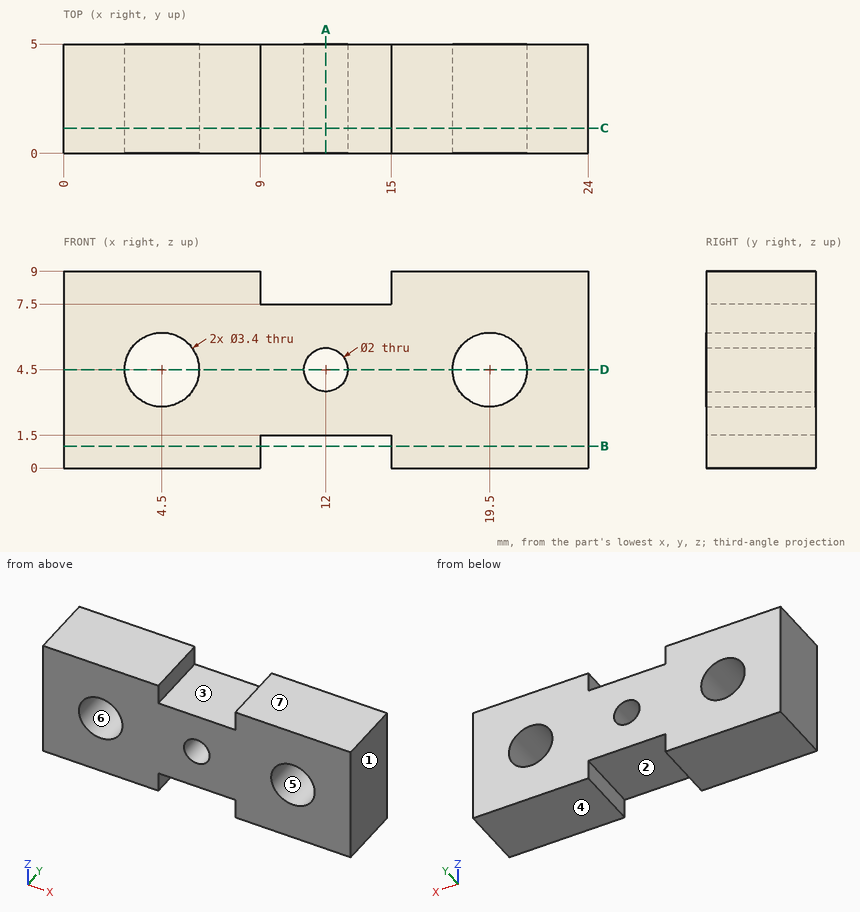
Design review of the part shown in the three views and the two pictorial views. Dimensions are in mm from the part's minimum x, y and z. A direction names the side the tool comes from. Coordinates: 2 decimals unless noted, no trailing zeros. Order: outer loops, then holes, each group sorted by start corner. A loop starts at its lowest first (then second) coordinate and runs counter-clockwise, first axis right, second up.
1) Take a section at A-A, the plane x = 12. Give the boundary of the cut face in (y, z), and give its area (3 significant figures).
2) Wall thickness on line 1 along X through (y, z) = (1.25, 4.5); line 2 along Z through (x, y) = (4.5, 2.85); line 3 along X through (y, z) = (1, 3.75): over which ranges is each line inside the solid? List them lowest first.
3) Clearance check with a flat-ended pin moving along its axis: pin 1 (1.5 mm diameter, centred on x = 12, y = 1.5, fed in from -Z). State where the tip first meets the part, or that it passes through.
4) Take a section at C-C, the plane y = 1.15. Give the boundary of the cut face in (x, z), and give its area (3 significant figures).
5) Take a section at B-B, the plane z = 1. Give the boundary of the cut face in (x, y), and give its area (3 significant figures).
6) Mouldability with a two-part tool opening along Z and no side actions: class the marked faces 4, 5, 6 and 7 as +Z half, -Z half, draft (parallel to the pull), parting line (faces both ways), or undercut.
7) For the marked faces 1, 2 and 3, list the 3-axis set-ups (+Z, -Z, +X, -X, +Y, -Y) from which the entire face can be reached by the end or side of a thin tool; tool diameter is ignored.
8) Take a section at D-D, the plane z = 4.5. Give the boundary of the cut face in (x, y), and give its area (3 significant figures).
Returned:
1. outline: (0, 1.5) - (5, 1.5) - (5, 3.5) - (0, 3.5) - close; (0, 5.5) - (5, 5.5) - (5, 7.5) - (0, 7.5) - close
1. area: 20.0 mm2
2. line 1: x = 0 to 2.8, 6.2 to 11, 13 to 17.8, 21.2 to 24
2. line 2: z = 0 to 2.8, 6.2 to 9
2. line 3: x = 0 to 2.97, 6.03 to 11.34, 12.66 to 17.97, 21.03 to 24
3. pin 1: stops at z = 1.5
4. outline: (0, 0) - (9, 0) - (9, 1.5) - (15, 1.5) - (15, 0) - (24, 0) - (24, 9) - (15, 9) - (15, 7.5) - (9, 7.5) - (9, 9) - (0, 9) - close; hole circle Ø3.4 at (4.5, 4.5); hole circle Ø2 at (12, 4.5); hole circle Ø3.4 at (19.5, 4.5)
4. area: 177 mm2
5. outline: (0, 0) - (9, 0) - (9, 5) - (0, 5) - close; (15, 0) - (24, 0) - (24, 5) - (15, 5) - close
5. area: 90.0 mm2
6. face 4: -Z half
6. face 5: undercut
6. face 6: undercut
6. face 7: +Z half
7. face 1: +Z, -Z, +X, +Y, -Y
7. face 2: -Z, +Y, -Y
7. face 3: +Z, +Y, -Y
8. outline: (0, 0) - (2.8, 0) - (2.8, 5) - (0, 5) - close; (6.2, 0) - (11, 0) - (11, 5) - (6.2, 5) - close; (13, 0) - (17.8, 0) - (17.8, 5) - (13, 5) - close; (21.2, 0) - (24, 0) - (24, 5) - (21.2, 5) - close
8. area: 76.0 mm2
